Check sheet for the modelled part. Datum: model origin and axes. Units: mm. A direction names the side the tool comes from. Round coordinates to 2 decimals unless told otherwise and drop trailing zeros. Order: outer loops, then holes, each group sorted by start corner. A loop starts at its lowest first (then second) coordinate and runs counter-clockwise, first axis right, second up.
Q1. Cross-section at C-C on y = -20. Record the cut outline in (x, z).
Q2. Depth check by flat-ended pin: P1, Ø6, axis at x = -8, z = 4, coming from the +Y side; P2, Ø3, axis at x = -20, y = 0, coming from the +Z side; P3, Ø18.5, axis at x = 0, y = 0, coming from the +Z side. Enter the tip coordinate at first touch or a pass-through.
Q3. Mould release check, pull along X, two halves, no side actions. Record for faces 1 (the cylindrical face through (-1.756, -7.907, 3.448)), 2 (the flat face through (19.8, 0, 2)), 3 (the cylindrical face through (-11.366, 10.492, 8.529)), 4 (the flat face through (4, 10, 6.8)): +X half, -X half, draft (parallel to the pull), parting line (faces both ways), or undercut.
Q4. Scan lines: probe 1 along Y at (x, z) = (0, 1.8); probe 2 along Z at (x, y) = (-14, 7); probe 3 along X at (y, z) = (-1, 0.5). Record each from-to range of solid material in increasing order.
Q5. Cross-section at A-A on y = 0. Record the cut outline in (x, z).
Q6. Cross-section at D-D on z = 1.5. Record the cut outline in (x, y), then the cut area to 3 significant figures.
Q7. Set-up check for faces 5 (the cylindrical face through (-10.79, 7.88, 5.32)), 6 (the cylindrical face through (0.27, 21.22, 1.87)): record each of +Z, -Z, +X, -X, +Y, -Y from which the full face is reachable in a straight line by a thin tool's end or side.
Q8. Cross-section at B-B on x = 0. Record the cut outline in (y, z), then the cut area to 3 significant figures.
from build123d import *

# Parameters (mm, degrees)
SKETCH_1_R          = 22.5
SKETCH_1_R_2        = 1.25
EXTRUDE_1_DEPTH     = 3.8
SKETCH_2_R          = 17.5
EXTRUDE_2_DEPTH     = 3
SKETCH_3_R          = 2
EXTRUDE_3_DEPTH     = 3.5
FILLET_1_R          = 0.5
FILLET_2_R          = 0.25
CUT_EXTRUDE_1_DEPTH = 3
SKETCH_5_R          = 8.1
CUT_EXTRUDE_2_DEPTH = 11
SKETCH_6_W          = 10.283159463
SKETCH_6_H          = 33.988548121
CUT_EXTRUDE_3_DEPTH = 17


with BuildPart() as part:
    # 草图1 → 凸台-拉伸1 (new body)
    with BuildSketch(Plane.XY):
        with Locations(Location((0, 0, 0), (0, 0, 180))):
            Circle(SKETCH_1_R)
        with Locations(Location((0, 20, 0), (0, 0, 180))):
            Circle(SKETCH_1_R_2, mode=Mode.SUBTRACT)
        with Locations(Location((0, -20, 0), (0, 0, 180))):
            Circle(SKETCH_1_R_2, mode=Mode.SUBTRACT)
        with Locations(Location((-20, 0, 0), (0, 0, 180))):
            Circle(SKETCH_1_R_2, mode=Mode.SUBTRACT)
    extrude(amount=EXTRUDE_1_DEPTH)

    # 草图2 → 凸台-拉伸2 (add)
    with BuildSketch(Plane.XY.offset(3.8)):
        Circle(SKETCH_2_R)
    extrude(amount=EXTRUDE_2_DEPTH)

    # 草图3 → 凸台-拉伸3 (add)
    with BuildSketch(Plane.XY.offset(6.8)):
        with Locations((-9.367828489, 10.404027557)):
            Circle(SKETCH_3_R)
    extrude(amount=EXTRUDE_3_DEPTH)

    # 圆角1
    fillet_1_edges = [part.edges().sort_by_distance(p)[0] for p in [
        (-17.5, 0, 6.8),
    ]]
    fillet(fillet_1_edges, radius=FILLET_1_R)

    # 圆角2
    fillet_2_edges = [part.edges().sort_by_distance(p)[0] for p in [
        (-11.367828489, 10.404027557, 6.8),
        (-11.367828489, 10.404027557, 10.3),
    ]]
    fillet(fillet_2_edges, radius=FILLET_2_R)

    # 草图4 → 切除-拉伸1 (cut)
    with BuildSketch(Plane.XY.offset(6.8)):
        with BuildLine():
            ThreePointArc((-16.962482908, 6.022804462), (-8.539705078, -15.845297005), (14.357267915, -10.856742514))
            ThreePointArc((14.357267915, -10.856742514), (13.579373382, -5.253629085), (7.976259953, -6.031523619))
            ThreePointArc((7.976259953, -6.031523619), (-4.744280599, -8.802942781), (-9.423601616, 3.346002479))
            ThreePointArc((-9.423601616, 3.346002479), (-11.85464127, 8.453844117), (-16.962482908, 6.022804462))
        make_face()
    extrude(amount=-CUT_EXTRUDE_1_DEPTH, mode=Mode.SUBTRACT)

    # 草图5 → 切除-拉伸2 (cut)
    with BuildSketch(Plane.XY.offset(6.8)):
        Circle(SKETCH_5_R)
    extrude(amount=-CUT_EXTRUDE_2_DEPTH, mode=Mode.SUBTRACT)

    # 草图6 → 切除-拉伸3 (cut)
    with BuildSketch(Plane.XY.offset(3.8)):
        with Locations((24.941579731, -0.947133109)):
            Rectangle(SKETCH_6_W, SKETCH_6_H)
    extrude(amount=-CUT_EXTRUDE_3_DEPTH, mode=Mode.SUBTRACT)


solid = part.part
Results found:
1. outline: (-10.31, 0) - (-1.25, 0) - (-1.25, 3.8) - (-10.31, 3.8) - close; (1.25, 0) - (10.31, 0) - (10.31, 3.8) - (1.25, 3.8) - close
2. P1: stops at y = 21.94
2. P2: stops at z = 3.8
2. P3: stops at z = 6.8
3. face 1: undercut
3. face 2: +X half
3. face 3: parting line
3. face 4: draft
4. probe 1: y = -22.5 to -21.25, -18.75 to -8.1, 8.1 to 18.75, 21.25 to 22.5
4. probe 2: z = 0 to 3.8
4. probe 3: x = -22.48 to -20.75, -19.25 to -8.04, 8.04 to 19.8
5. outline: (-22.5, 0) - (-21.25, 0) - (-21.25, 3.8) - (-22.5, 3.8) - close; (-18.75, 0) - (-8.1, 0) - (-8.1, 6.8) - (-10, 6.8) - (-10, 3.8) - (-18.75, 3.8) - close; (8.1, 0) - (19.8, 0) - (19.8, 3.8) - (17.5, 3.8) - (17.5, 6.3) arc R0.5 ccw to (17, 6.8) - (8.1, 6.8) - close
6. outline: (19.8, -10.69) - (19.8, 10.69) arc R22.5 ccw (long way) to start; hole circle Ø2.5 at (-20, 0); hole circle Ø16.2 at (0, 0); hole circle Ø2.5 at (0, -20); hole circle Ø2.5 at (0, 20)
6. area: 1,330 mm2
7. face 5: +Z
7. face 6: +Z, -Z
8. outline: (-22.5, 0) - (-21.25, 0) - (-21.25, 3.8) - (-22.5, 3.8) - close; (-18.75, 0) - (-8.1, 0) - (-8.1, 6.8) - (-10, 6.8) - (-10, 3.8) - (-18.75, 3.8) - close; (8.1, 0) - (18.75, 0) - (18.75, 3.8) - (17.5, 3.8) - (17.5, 6.3) arc R0.5 ccw to (17, 6.8) - (8.1, 6.8) - close; (21.25, 0) - (22.5, 0) - (22.5, 3.8) - (21.25, 3.8) - close
8. area: 124 mm2
